The model under review builds one solid part; all positions refer to its coordinate system, in mm. A direction names the side the tool comes from. Round coordinates to 2 decimals unless told otherwise and drop trailing zeros. Write each loop counter-clockwise with the first axis right and the second up, starting at its lowest first coordinate (ties: lowest second). Pieces come first, ordered by that corner, then holes. Notation, with made-up numbers: (-25.75, -12.5) - (22.25, -12.5) arc R30 ccw to (22.25, 14.5) - close; hole circle Ø6 at (-33.75, -10.75). An arc over 180 degrees is marked (long way). Write each question's results on one line, items separated by ' | '.
```python
from build123d import *

# Parameters (mm, degrees)
SKETCH1_W           = 150
SKETCH1_H           = 80
BOSS_EXTRUDE1_DEPTH = 3
SKETCH2_W           = 3
SKETCH2_H           = 60
CUT_EXTRUDE1_DEPTH  = 10


with BuildPart() as part:
    # Sketch1 → Boss-Extrude1 (new body)
    with BuildSketch(Plane(origin=(0, 0, 0), x_dir=(1, 0, 0), z_dir=(0, 1, 0))):
        with Locations((75, 40)):
            Rectangle(SKETCH1_W, SKETCH1_H)
    extrude(amount=BOSS_EXTRUDE1_DEPTH)

    # Sketch2 → Cut-Extrude1 (cut)
    with BuildSketch(Plane(origin=(0, 0, 0), x_dir=(1, 0, 0), z_dir=(0, 1, 0))):
        with Locations((11.5, 40)):
            Rectangle(SKETCH2_W, SKETCH2_H)
        with Locations((138.5, 40)):
            Rectangle(SKETCH2_W, SKETCH2_H)
    extrude(amount=CUT_EXTRUDE1_DEPTH, mode=Mode.SUBTRACT)


solid = part.part
```
Q1. Tool access review of faces 1 (the flat face through (150, 1, -39)), 2 (the flat face through (137, 1, -40)): name each direction out of +Z, -Z, +X, -X, +Y, -Y from which nothing blocks a thin tool from reaching the whole face with its end or side.
Evaluation:
face 1: +Z, -Z, +X, +Y, -Y | face 2: +Y, -Y
Q2. The part is to be moulded in two halves that separate along Z. For faces 3 (the flat face through (10, 1, -40)), 4 (the flat face through (74, 0, -41)), 5 (the flat face through (74, 1, -80)), 6 (the flat face through (140, 1, -40)), say which applies: released by +Z, released by -Z, zero draft, split by the parting line, or undercut.
Evaluation:
face 3: undercut | face 4: zero draft | face 5: released by -Z | face 6: undercut
Q3. For probe 1 along X at (y, z) = (2.65, -43.5); probe 2 along Z at (x, y) = (139.5, 0.75), list the stretches that pass through material, from the lowest coordinate up.
Evaluation:
probe 1: x = 0 to 10, 13 to 137, 140 to 150 | probe 2: z = -80 to -70, -10 to 0
Q4. We need section A-A (y = 1.25). State the section outline as (x, z) points.
Evaluation:
outline: (0, -80) - (150, -80) - (150, 0) - (0, 0) - close; hole (10, -70) - (13, -70) - (13, -10) - (10, -10) - close; hole (137, -70) - (140, -70) - (140, -10) - (137, -10) - close
Q5. We need section B-B (z = -21). State the section outline as (x, y) points.
Evaluation:
outline: (0, 0) - (10, 0) - (10, 3) - (0, 3) - close; (13, 0) - (137, 0) - (137, 3) - (13, 3) - close; (140, 0) - (150, 0) - (150, 3) - (140, 3) - close
